The model under review builds one solid part; all positions refer to its coordinate system, in mm. A direction names the side the tool comes from. Round coordinates to 2 decimals unless told otherwise and drop trailing zeros. Write each loop counter-clockwise with the first axis right and the second up, starting at its lowest first coordinate (ties: lowest second). Pieces come first, ordered by that corner, then holes.
Item 1: Draft analysis for pull direction X (two halves, no side actions). For faces 1 (the face through (2.097, -0.009, 0.024)), 2 (the face through (0, 9, 1)), 3 (the face through (8.43, -8.4, 1.18)), state which applies: +X half, -X half, draft (parallel to the pull), parting line (faces both ways), or undercut.
Item 2: Clearance check with flat-ended pins moving along their axes: pin 1 Ø6 at (x, y) = (7, 6) entering from -Z; pin 2 Ø10 at (x, y) = (-0.5, 0.5) entering from +Z; pin 3 Ø0.7 at (x, z) = (1, -0.5) entering from +Y. State where each tip first meets the part, or that it passes through.
Item 3: Machinability: for faces 4 (the face through (0.63, -1, 0)), 5 (the face through (-8.43, -8.4, 1.18)), which of the approach directions +Z, -Z, +X, -X, +Y, -Y give a long, thin tool a straight path to every point of the face, cutting with its end or side? Answer none if there is none.
Item 4: To check wall thickness, follow L1, parallel to X at y = 5.75, z = 0.45; L2, parallel to Y at x = 5.25, z = 0.75; L3, parallel to Y at x = -2.5, z = 1.45. State the ranges of each line that lie inside material, in increasing order.
Item 5: Add section A-A (z = -0.4). Give the boundary of the cut face in (x, y).
```python
from build123d import *

# Parameters (mm, degrees)
SKETCH_W        = 9
SKETCH_H        = 18
PAD_DEPTH       = 2.7
PAD001_DEPTH    = 9
POCKET_DEPTH    = 10
POCKET001_DEPTH = 1.7
PAD002_DEPTH    = 3.4


with BuildPart() as part:
    # Sketch → Pad (new body)
    with BuildSketch(Plane.XY):
        with Locations((-4.5, 0)):
            Rectangle(SKETCH_W, SKETCH_H)
    extrude(amount=PAD_DEPTH)

    # Sketch001 → Pad001 (join, symmetric)
    with BuildSketch(Plane.XZ):
        with BuildLine():
            Line((-9, 2.7), (0, 2.7))
            Line((0, 2.7), (0, 3))
            add(Edge.make_bspline(
                [(0, 3), (-2.554918, 2.91153), (-5.658926, 3.478662), (-7.63445, 4.400123), (-9, 3.5)],
                knots=[0, 0, 0, 0, 0.5, 1, 1, 1, 1], degree=3))
            Line((-9, 3.5), (-9, 2.7))
        make_face()
    extrude(amount=PAD001_DEPTH, both=True)

    # Sketch002 → Pocket (cut)
    with BuildSketch(Plane.XY):
        with BuildLine():
            ThreePointArc((-7, 9), (-8.414214, 8.414214), (-9, 7))
            Line((-9, 7), (-10, 7))
            Line((-10, 7), (-10, 10))
            Line((-10, 10), (-7, 10))
            Line((-7, 10), (-7, 9))
        make_face()
        with BuildLine():
            ThreePointArc((-9, -7), (-8.414214, -8.414214), (-7, -9))
            Line((-7, -9), (-7, -10))
            Line((-10, -10), (-7, -10))
            Line((-10, -7), (-10, -10))
            Line((-9, -7), (-10, -7))
        make_face()
    extrude(amount=POCKET_DEPTH, mode=Mode.SUBTRACT)

    # Sketch003 → Pocket001 (cut)
    with BuildSketch(Plane.XY):
        with BuildLine():
            Line((0, 7.8), (-6.25, 7.8))
            ThreePointArc((-6.25, 7.8), (-7.31066, 7.36066), (-7.75, 6.3))
            Line((-7.75, 6.3), (-7.75, -6.3))
            ThreePointArc((-7.75, -6.3), (-7.31066, -7.36066), (-6.25, -7.8))
            Line((-6.25, -7.8), (0, -7.8))
            Line((0, -7.8), (0, 0))
            Line((0, 0), (0, 7.8))
        make_face()
    extrude(amount=POCKET001_DEPTH, mode=Mode.SUBTRACT)

    # Sketch004 (on Face10 of Pocket001) → Pad002 (join)
    with BuildSketch(Plane(origin=(0, 0, 1.7), x_dir=(1, 0, 0), z_dir=(0, 0, -1))):
        with BuildLine():
            ThreePointArc((0, 2.75), (-2.75, 0), (0, -2.75))
            Line((0, -2.096879), (0, -2.75))
            ThreePointArc((-0.63, -2), (-0.318703, -2.072517), (0, -2.096879))
            Line((-0.63, -0.63), (-0.63, -2))
            Line((-2, -0.63), (-0.63, -0.63))
            ThreePointArc((-2, 0.63), (-2.096879, 0), (-2, -0.63))
            Line((-2, 0.63), (-0.63, 0.63))
            Line((-0.63, 0.63), (-0.63, 2))
            ThreePointArc((0, 2.096879), (-0.318703, 2.072517), (-0.63, 2))
            Line((0, 2.75), (0, 2.096879))
        make_face()
    extrude(amount=PAD002_DEPTH)

    # SubtractivePipe: sweep along a path in Sketch009
    with BuildLine(Plane(origin=(0, 0, 2.4), x_dir=(0, -1, 0), z_dir=(0, 0, 1))) as subtractivepipe_path:
        Line((-9, 0), (-9, -7))
        ThreePointArc((-9, -7), (-8.414214, -8.414214), (-7, -9))
        Line((-7, -9), (7, -9))
        ThreePointArc((7, -9), (8.414214, -8.414214), (9, -7))
        Line((9, -7), (9, 0))
    # Sketch008 → SubtractivePipe (sweep, cut)
    with BuildSketch(Plane.YZ):
        Polygon((-9, 2.4), (-7.5, 4.05), (-9, 4.05), align=None)
    sweep(path=subtractivepipe_path.line, mode=Mode.SUBTRACT)

    # Mirrored: part across YZ


with BuildPart() as part_1:
    add(part.part)
    add(part.part.mirror(Plane.YZ))


solid = part_1.part
```
Numbers:
1. face 1: undercut
1. face 2: draft
1. face 3: +X half
2. pin 1: stops at z = 0
2. pin 2: stops at z = 3.6
2. pin 3: stops at y = 2.67
3. face 4: -Z
3. face 5: +Z, -Z, -X, -Y
4. L1: x = -9 to -7.75, 7.75 to 9
4. L2: y = -9 to -7.8, 7.8 to 9
4. L3: y = -9 to -7.8, -1.15 to 1.15, 7.8 to 9
5. outline: circle Ø5.5 at (0, 0); hole (-2, -0.63) - (-0.63, -0.63) - (-0.63, -2) arc R2.1 ccw to (0, -2.1) arc R2.1 ccw to (0.63, -2) - (0.63, -0.63) - (2, -0.63) arc R2.1 ccw to (2, 0.63) - (0.63, 0.63) - (0.63, 2) arc R2.1 ccw to (0, 2.1) arc R2.1 ccw to (-0.63, 2) - (-0.63, 0.63) - (-2, 0.63) arc R2.1 ccw to start
